```python
from build123d import *

# Parameters (mm, degrees)
SKETCH1_W           = 12.2
SKETCH1_H           = 10
BOSS_EXTRUDE1_DEPTH = 10
SKETCH2_R           = 2.125
CUT_EXTRUDE1_DEPTH  = 12.2
SKETCH3_W           = 15
SKETCH3_H           = 10
BOSS_EXTRUDE2_DEPTH = 5
SKETCH4_R           = 4
BOSS_EXTRUDE3_DEPTH = 254


with BuildPart() as part:
    # Sketch1 → Boss-Extrude1 (new body)
    with BuildSketch(Plane.XY):
        Rectangle(SKETCH1_W, SKETCH1_H)
    extrude(amount=BOSS_EXTRUDE1_DEPTH)

    # Sketch2 → Cut-Extrude1 (cut)
    with BuildSketch(Plane.ZY.offset(6.1)):
        with Locations((4.889205296, 0)):
            Circle(SKETCH2_R)
        with BuildLine():
            Line((4.889205296, 3.125), (0, 3.125))
            Line((0, 3.125), (0, 5))
            Line((0, 5), (10, 5))
            Line((10, 5), (10, -5))
            Line((10, -5), (0, -5))
            Line((0, -5), (0, -3.125))
            Line((0, -3.125), (4.889205296, -3.125))
            ThreePointArc((4.889205296, -3.125), (8.014205296, 0), (4.889205296, 3.125))
        make_face()
    extrude(amount=-CUT_EXTRUDE1_DEPTH, mode=Mode.SUBTRACT)

    # Sketch3 → Boss-Extrude2 (add)
    with BuildSketch(Plane(origin=(0, 0, 0), x_dir=(-1, 0, 0), z_dir=(0, 0, -1))):
        Rectangle(SKETCH3_W, SKETCH3_H)
    extrude(amount=BOSS_EXTRUDE2_DEPTH)

    # Sketch4 → Boss-Extrude3 (add)
    with BuildSketch(Plane(origin=(0, 0, -5), x_dir=(-1, 0, 0), z_dir=(0, 0, -1))):
        Circle(SKETCH4_R)
    extrude(amount=BOSS_EXTRUDE3_DEPTH)


solid = part.part
```
For this review, take the finished solid that the model builds, in its own axes (mm). A direction names the side the tool comes from. Coordinates: 2 decimals unless noted, no trailing zeros. Write each loop counter-clockwise with the first axis right and the second up, starting at its lowest first coordinate (ties: lowest second). Pieces come first, ordered by that corner, then holes.
(1) Add section B-B on x = 0. Give the boundary of the cut face in (y, z) (3 decimals).
(2) Wall thickness on probe 1 along Z at (x, y) = (2.25, 4); probe 2 along Y at (x, z) = (-0.5, -209.5); probe 3 along X at (y, z) = (-2.5, -117.5): over which ranges is each line inside the solid? List them lowest first.
(3) Tool access review of faces 1 (the face through (0, -3.125, 2)), 2 (the face through (-6.1, 0, 2)), 3 (the face through (6.1, 0, 2)), 4 (the face through (0, 0, -259)), 5 (the face through (0.867, -3.905, -130.222)): name each direction out of +Z, -Z, +X, -X, +Y, -Y from which nothing blocks a thin tool from reaching the whole face with its end or side.
(4) For pin 1 Ø5.5 at (x, z) = (-2, 1.5) entering from +Y; pin 2 Ø4 at (x, z) = (2, -143) entering from +Y; pin 3 Ø4 at (x, z) = (3, -94) entering from -Y; pin 4 Ø1.5 at (x, z) = (-2, -203) entering from +Y, all flat-tipped, find the tip position at first contact; note any pin that passes through.
(5) Add section A-A on y = 0. Give the boundary of the cut face in (x, z), then the cut area to 3 significant figures.
(6) The part is to be moulded in two halves that separate along Y. For faces 6 (the face through (-0.085, 0.093, 2.766)), 7 (the face through (-7.5, 0, -2)), 8 (the face through (0, 3.125, 2)), say which applies: +Y half, -Y half, draft (parallel to the pull), parting line (faces both ways), or undercut.
(7) Add section C-C on z = -53.5. Give the boundary of the cut face in (x, y), then the cut area to 3 significant figures.
Answer sheet:
1. outline: (-5, -5) - (-4, -5) - (-4, -259) - (4, -259) - (4, -5) - (5, -5) - (5, 0) - (3.125, 0) - (3.125, 4.889) arc R3.125 ccw to (-3.125, 4.889) - (-3.125, 0) - (-5, 0) - close; hole circle Ø4.25 at (0, 4.889)
2. probe 1: z = -5 to 0
2. probe 2: y = -3.97 to 3.97
2. probe 3: x = -3.12 to 3.12
3. face 1: +Z, +X, -X, -Y
3. face 2: +Z, -X, +Y, -Y
3. face 3: +Z, +X, +Y, -Y
3. face 4: -Z, +X, -X, +Y, -Y
3. face 5: -Z
4. pin 1: stops at y = 5
4. pin 2: stops at y = 4
4. pin 3: stops at y = -3.87
4. pin 4: stops at y = 3.8
5. outline: (-7.5, -5) - (-4, -5) - (-4, -259) - (4, -259) - (4, -5) - (7.5, -5) - (7.5, 0) - (6.1, 0) - (6.1, 2.76) - (-6.1, 2.76) - (-6.1, 0) - (-7.5, 0) - close; (-6.1, 7.01) - (6.1, 7.01) - (6.1, 8.01) - (-6.1, 8.01) - close
5. area: 2,150 mm2
6. face 6: undercut
6. face 7: draft
6. face 8: +Y half
7. outline: circle Ø8 at (0, 0)
7. area: 50.3 mm2
